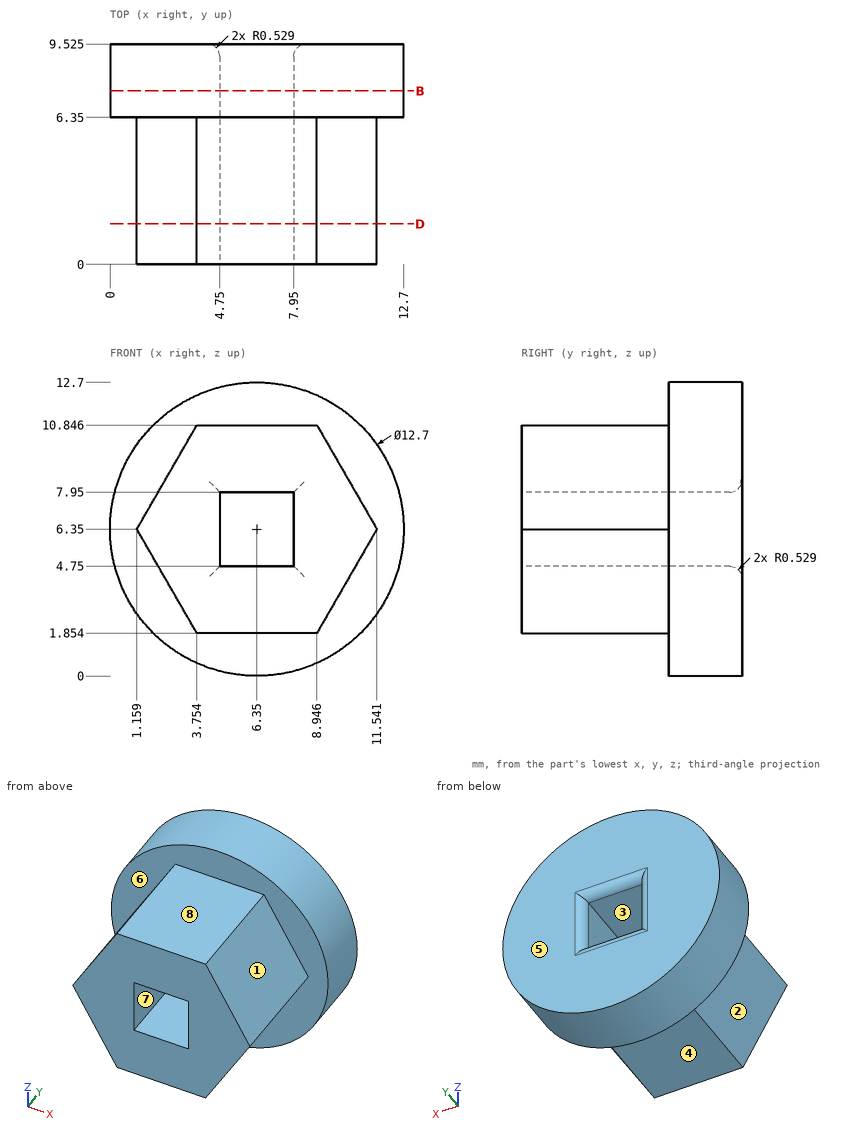
Job drawing, mm, ordinate dimensions from the low corner. One solid piece. A direction names the side the tool comes from. Give positions to 0.01 mm unless a question says otherwise; leave off trailing zeros. Loops run counter-clockwise (first coordinate to the right, second up) from the corner with the lowest first, then second, coordinate; pieces in that order, holes last. Notation, with made-up numbers: (38, 16) -> (59, 16) arc R28 ccw to (59, 48) -> close; hole circle Ø11 at (34.5, -39.75). An arc over 180 degrees is marked (long way). Write each question's results on one line, items separated by ' | '.
(1) Cut at D-D on y = 1.75. List the corners of the cut face in (x, z).
Geometry results:
outline: (1.16, 6.35) -> (3.75, 1.85) -> (8.95, 1.85) -> (11.54, 6.35) -> (8.95, 10.85) -> (3.75, 10.85) -> close; hole (4.75, 4.75) -> (7.95, 4.75) -> (7.95, 7.95) -> (4.75, 7.95) -> close
(2) Tool access for the marked faces 5, 6, 7 and 8: list every direction of +Z, -Z, +X, -X, +Y, -Y with a clear straight run to the whole face (end or side of a thin tool).
Geometry results:
face 5: +Z, -Z, +X, -X, +Y | face 6: -Y | face 7: +Y, -Y | face 8: +Z, +X, -X, -Y
(3) Flat gauge pins, fed straight in: pin 1 Ø1 at (y, z) = (2.5, 7) entering from -X (1 decimal); pin 2 Ø2.5 at (x, y) = (5.5, 4) entering from -Z; pin 3 Ø1.6 at (x, y) = (5.5, 2) entering from +Z. Where does each tip first touch, or does it go through?
Geometry results:
pin 1: stops at x = 1.2 | pin 2: stops at z = 1.85 | pin 3: stops at z = 10.85
(4) Cut at B-B on y = 7.5. List the corners of the cut face in (x, z).
Geometry results:
outline: circle Ø12.7 at (6.35, 6.35); hole (4.75, 4.75) -> (7.95, 4.75) -> (7.95, 7.95) -> (4.75, 7.95) -> close
(5) Pull direction X, two halves, no side cores. Call the marked faces 1, 2, 3 and 4: released by +X, released by -X, zero draft, split by the parting line, or undercut.
Geometry results:
face 1: released by +X | face 2: released by -X | face 3: undercut | face 4: zero draft
(6) Probe line 1 along Z through (x, y) = (7, 0.5); line 2 along X through (y, z) = (2.75, 6.25); line 3 along X through (y, z) = (2.5, 6.75). List the from-to ranges inside material, lowest first.
Geometry results:
line 1: z = 1.85 to 4.75, 7.95 to 10.85 | line 2: x = 1.22 to 4.75, 7.95 to 11.48 | line 3: x = 1.39 to 4.75, 7.95 to 11.31
